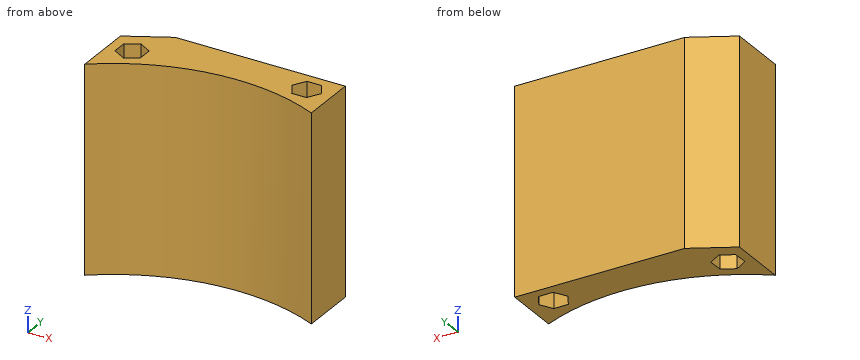
```python
from build123d import *

# Parameters (mm, degrees)
BOSS_EXTRUDE1_DEPTH = 65
CUT_EXTRUDE1_DEPTH  = 5
CUT_EXTRUDE2_DEPTH  = 5
SKETCH4_R           = 2.1
CUT_EXTRUDE3_DEPTH  = 10
SKETCH5_R           = 2.1
CUT_EXTRUDE4_DEPTH  = 10


with BuildPart() as part:
    # Sketch1 → Boss-Extrude1 (new body)
    with BuildSketch(Plane.XY):
        with BuildLine():
            Line((-26.885, 0), (26.885, 0))
            Line((26.885, 0), (26.885, -17.820638944))
            ThreePointArc((26.885, -17.820638944), (-7.666811739, -12.453737538), (-40, -25.76524617))
            Line((-40, -25.76524617), (-40, -7))
            Line((-40, -7), (-26.885, 0))
        make_face()
    extrude(amount=BOSS_EXTRUDE1_DEPTH)

    # Sketch2 → Cut-Extrude1 (cut)
    with BuildSketch(Plane.XY.offset(65)):
        Polygon((-32.94236854, -17.234485077), (-28.94236854, -14.925084), (-28.94236854, -10.306281847), (-32.94236854, -7.99688077), (-36.94236854, -10.306281847), (-36.94236854, -14.925084), align=None)
        Polygon((14.266197846, -7), (16.575598923, -11), (21.194401077, -11), (23.503802154, -7), (21.194401077, -3), (16.575598923, -3), align=None)
    extrude(amount=-CUT_EXTRUDE1_DEPTH, mode=Mode.SUBTRACT)

    # Sketch3 → Cut-Extrude2 (cut)
    with BuildSketch(Plane(origin=(0, 0, 0), x_dir=(-1, 0, 0), z_dir=(0, 0, -1))):
        Polygon((28.861855536, -10.451717361), (29.028062888, -15.067528064), (33.108575892, -17.231493627), (37.022881544, -14.779648487), (36.856674193, -10.163837783), (32.776161189, -7.99987222), align=None)
        Polygon((-16.5261006, -10.971010823), (-14.266554049, -6.942638606), (-16.625453449, -2.971627783), (-21.2438994, -3.028989177), (-23.503445951, -7.057361394), (-21.144546551, -11.028372217), align=None)
    extrude(amount=-CUT_EXTRUDE2_DEPTH, mode=Mode.SUBTRACT)

    # Sketch4 → Cut-Extrude3 (cut)
    with BuildSketch(Plane(origin=(0, 0, 5), x_dir=(-1, 0, 0), z_dir=(0, 0, -1))):
        with Locations((32.94236854, -12.615682924)):
            Circle(SKETCH4_R)
        with Locations((-18.885, -7)):
            Circle(SKETCH4_R)
    extrude(amount=-CUT_EXTRUDE3_DEPTH, mode=Mode.SUBTRACT)

    # Sketch5 → Cut-Extrude4 (cut)
    with BuildSketch(Plane.XY.offset(60)):
        with Locations((-32.94236854, -12.615682924)):
            Circle(SKETCH5_R)
        with Locations((18.885, -7)):
            Circle(SKETCH5_R)
    extrude(amount=-CUT_EXTRUDE4_DEPTH, mode=Mode.SUBTRACT)


solid = part.part
```
CAD build for the part. Positions are in the model's coordinates, mm. Round coordinates to 2 decimals unless told otherwise and drop trailing zeros. Loops run counter-clockwise (first coordinate to the right, second up) from the corner with the lowest first, then second, coordinate; pieces in that order, holes last. Notation, with made-up numbers: M -24.75,33.25 L 7.25,33.25 A17 ccw 7.25,51.25 Z; hole C -9.75,12.5 d4. An arc over 180 degrees is marked long. Use a Markdown table: item, result. Add a question column.
(1) Drill centre lines: line 1 (X direction, y = -4, z = 3.5) (3 decimals); line 2 (Y direction, x = -34.5, z = 13); line 3 (Y direction, x = 18.5, z = 4). Where is each one in solid material? Low to high.
(2) Cut at C-C (y = -23.25). Give the cut face in (x, z), and give its area (3 significant figures).
(3) Cut at B-B (z = 14). Give the cut face in (x, y) (3 decimals), and give its area (3 significant figures).
(4) Flat gauge pins, fed straight in: pin 1 (5 mm diameter, centred on x = -33, z = 35.5, fed in from +Y); pin 2 (5.5 mm diameter, centred on x = 18.885, y = -7, fed in from -Z); pin 3 (2.5 mm diameter, centred on x = -32.94, y = -12.62, fed in from +Z). Where does each tip first touch, or does it go through?
(5) Cut at D-D (x = -13). Give the cut face in (y, z).
(6) Cut at A-A (z = 41). Give the cut face in (x, y) (3 decimals), and give its area (3 significant figures).
Geometry says:
| question | item | result |
|---|---|---|
| 1 | line 1 | x = -34.379 to 16.015, 21.789 to 26.885 |
| 1 | line 2 | y = -21.91 to -14.02, -11.21 to -4.06 |
| 1 | line 3 | y = -14.69 to -11, -2.99 to 0 |
| 2 | outline | M -40,0 L -36.55,0 L -36.55,65 L -40,65 Z |
| 2 | area | 224 mm² |
| 3 | outline | M -40,-25.765 A65 cw 26.885,-17.821 L 26.885,0 L -26.885,0 L -40,-7 Z; hole C -32.942,-12.616 d4.2; hole C 18.885,-7 d4.2 |
| 3 | area | 955 mm² |
| 4 | pin 1 | stops at y = -1.93 |
| 4 | pin 2 | stops at z = 5 |
| 4 | pin 3 | stops at z = 50 |
| 5 | outline | M -13.31,0 L 0,0 L 0,65 L -13.31,65 Z |
| 6 | outline | M -40,-25.765 A65 cw 26.885,-17.821 L 26.885,0 L -26.885,0 L -40,-7 Z |
| 6 | area | 983 mm² |
